```python
from build123d import *

# Parameters (mm, degrees)
F0_W     = 35
F0_H     = 15
F1_DEPTH = 17
F2_W     = 35
F2_H     = 4.99
F3_DEPTH = 20
F5_DEPTH = 13
F7_DEPTH = 25
F8_W     = 5
F8_H     = 5
F9_DEPTH = 3
F10_R    = 4


with BuildPart() as f1:
    # F0 (on Front) → F1 (new body)
    with BuildSketch(Plane.XZ):
        with Locations((-4.829492, -4.074684)):
            Rectangle(F0_W, F0_H)
    extrude(amount=F1_DEPTH)

    # F2 (on face) → F3 (join)
    with BuildSketch(Plane.XZ.offset(17)):
        with Locations((-4.829492, 0.930316)):
            Rectangle(F2_W, F2_H)
    extrude(amount=F3_DEPTH)

    # F4 (on face) → F5 (cut)
    with BuildSketch(Plane.XZ.offset(17)):
        Polygon((-11.329492, -7.574684), (-4.829492, -7.574684), (1.670508, -7.574684), (1.670508, -1.574684), (-11.329492, -1.574684), align=None)
    extrude(amount=-F5_DEPTH, mode=Mode.SUBTRACT)

    # F6 (on face) → F7 (cut)
    with BuildSketch(Plane(origin=(0, 0, -11.574684), x_dir=(1, 0, 0), z_dir=(0, 0, -1))):
        with BuildLine():
            ThreePointArc((-1.579492, 12.01), (-2.531395, 14.308097), (-4.829492, 15.26))
            ThreePointArc((-4.829492, 15.26), (-7.127589, 9.711903), (-1.579492, 12.01))
        make_face()
    extrude(amount=-F7_DEPTH, mode=Mode.SUBTRACT)

    # F8 (on face) → F9 (cut)
    with BuildSketch(Plane(origin=(0, 0, 0), x_dir=(-1, 0, 0), z_dir=(0, 1, 0))):
        with Locations((4.829492, -4.074684)):
            Rectangle(F8_W, F8_H)
    extrude(amount=-F9_DEPTH, mode=Mode.SUBTRACT)

    # F10
    f10_edges = [f1.edges().sort_by_distance(p)[0] for p in [
        (12.670508, -18.5, 3.425316),
        (-4.829492, -37, 3.425316),
        (-22.329492, -18.5, 3.425316),
        (-4.829492, 0, 3.425316),
        (-22.329492, 0, -4.074684),
        (12.670508, 0, -4.074684),
    ]]
    fillet(f10_edges, radius=F10_R)


solid = f1.part
```
Check sheet for the modelled part. Datum: model origin and axes. Units: mm. A direction names the side the tool comes from. Coordinates: 2 decimals unless noted, no trailing zeros. Loops run counter-clockwise (first coordinate to the right, second up) from the corner with the lowest first, then second, coordinate; pieces in that order, holes last. Notation, with made-up numbers: M -9,-29.75 L 41,-29.75 A27 cw 41,-6.75 Z; hole C 68,9.25 d1. An arc over 180 degrees is marked long. Answer as a JSON object with one key per item and string values.
1. Depth check by flat-ended pin: P1, Ø1.5, axis at y = -2, z = -4.5, coming from the -X side; P2, Ø5, axis at x = 2, z = -7.5, coming from the -Y side; P3, Ø10, axis at x = -1.5, y = -25, coming from the -Z side. Enter the tip coordinate at first touch or a pass-through.
Outcome:
{"P1": "x = -22.13", "P2": "y = -17", "P3": "z = -1.56"}
2. Access from +Z, -Z, +X, -X, +Y, -Y to the whole of each face (thin tool, end or side, straight path). Record for faces 1 (the flat face through (-5, -3, -4)), 2 (the flat face through (-5, -17, -8)), 3 (the flat face through (1.671, -11, -5)).
Outcome:
{"face 1": "+Y", "face 2": "-Z, +X, -X, -Y", "face 3": "-Y"}
3. Sectioned sample at C-C on x = -16. Record the cut outline in (y, z).
Outcome:
{"outline": "M -37,-1.56 L -17,-1.56 L -17,-11.57 L 0,-11.57 L 0,-0.57 A4 ccw -4,3.43 L -33,3.43 A4 ccw -37,-0.57 Z"}
4. Sectioned sample at B-B on y = -28. Record the cut outline in (x, z), and give its area (3 significant figures).
Outcome:
{"outline": "M -22.33,-1.56 L 12.67,-1.56 L 12.67,-0.57 A4 ccw 8.67,3.43 L -18.33,3.43 A4 ccw -22.33,-0.57 Z", "area": "168 mm²"}
5. Release check for a two-part mould opening along X. For faces 4 (the cylindrical face through (-21.19, -20.27, 2.22)), 5 (the cylindrical face through (-4.64, -1.2, 2.28)), 6 (the flat face through (-5, -1, -6.575)) record: pulls with the +X half, pulls with the -X half, needs draft (parallel to the pull), parting line crosses it, or undercut.
Outcome:
{"face 4": "pulls with the -X half", "face 5": "needs draft", "face 6": "undercut"}
6. Scan lines: L1, parallel to Y at x = -1.5, z = -2.25; L2, parallel to Z at x = 0, y = -11.5; L3, parallel to Y at x = -17, z = -4. Record each from-to range of solid material in increasing order. Write a range as from..to.
Outcome:
{"L1": "-4..0", "L2": "-11.57..-7.57, -1.57..3.43", "L3": "-17..0"}
7. Sectioned sample at A-A on x = -5.5. Count the separate pieces of the cut face and the enclosed holes in it, and give its area (3 significant figures).
Outcome:
{"separate pieces": "3", "enclosed holes": "0", "area": "198 mm²"}
